Here's the drawing with two shaded views (mm, measured from the low corner). I have some questions. Give positions to 0.01 mm unless a question says otherwise; leave off trailing zeros. Loops run counter-clockwise (first coordinate to the right, second up) from the corner with the lowest first, then second, coordinate; pieces in that order, holes last. Notation, with made-up numbers: M 10,51.5 L 58,51.5 A15 cw 58,79.5 Z; hole C 51,-40 d4. An arc over 180 degrees is marked long. Use a Markdown table: item, result. Add a question column.
1) Will these pins go through, and if not, where does the flat tip stop? pin 1 Ø12 at (x, y) = (83.5, 183.5) entering from -Z; pin 2 Ø1 at (x, z) = (51, 4.5) entering from +Y; pin 3 Ø0.6 at (y, z) = (157, 3.5) entering from +X; pin 4 Ø1.5 at (y, z) = (70.5, 4.5) entering from -X.
2) Suppose I cut it at A-A on x = 51.5. List the corners of the cut face in (y, z) for me, and give its area (3 significant figures).
3) Suppose I cut it at C-C on y = 61.5. List the corners of the cut face in (x, z) for me, and give its area (3 significant figures).
4) If I drill on line 1 along Y through (x, z) = (71, 3.4); line 2 along Y through (x, z) = (56.5, 0.5); line 3 along Y through (x, z) = (29, 3.1), over which ranges is the centre line in solid material (lowest first)? Write a range as [from, to].
5) Suppose I cut it at B-B on z = 1.25. List the corners of the cut face in (x, y) for me.
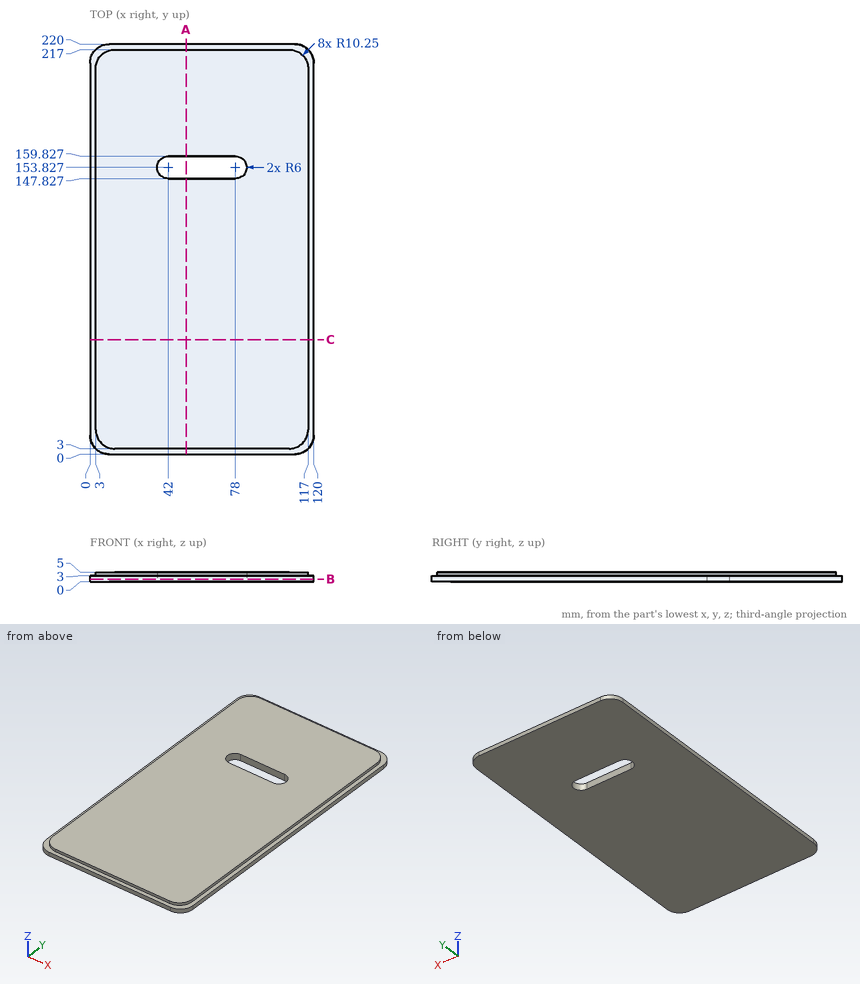
Answer block:
| question | item | result |
|---|---|---|
| 1 | pin 1 | stops at z = 0 |
| 1 | pin 2 | stops at y = 217 |
| 1 | pin 3 | stops at x = 117 |
| 1 | pin 4 | stops at x = 3 |
| 2 | outline | M 0,0 L 147.83,0 L 147.83,5 L 3,5 L 3,3 L 0,3 Z; M 159.83,0 L 220,0 L 220,3 L 217,3 L 217,5 L 159.83,5 Z |
| 2 | area | 1,030 mm^2 |
| 3 | outline | M 0,0 L 120,0 L 120,3 L 117,3 L 117,5 L 3,5 L 3,3 L 0,3 Z |
| 3 | area | 588 mm^2 |
| 4 | line 1 | y = [3, 147.83], [159.83, 217] |
| 4 | line 2 | y = [0, 147.83], [159.83, 220] |
| 4 | line 3 | y = [3, 217] |
| 5 | outline | M 0,10.25 A10.25 ccw 10.25,0 L 109.75,0 A10.25 ccw 120,10.25 L 120,209.75 A10.25 ccw 109.75,220 L 10.25,220 A10.25 ccw 0,209.75 Z; hole M 42,147.83 L 78,147.83 A6 ccw 78,159.83 L 42,159.83 A6 ccw Z |
